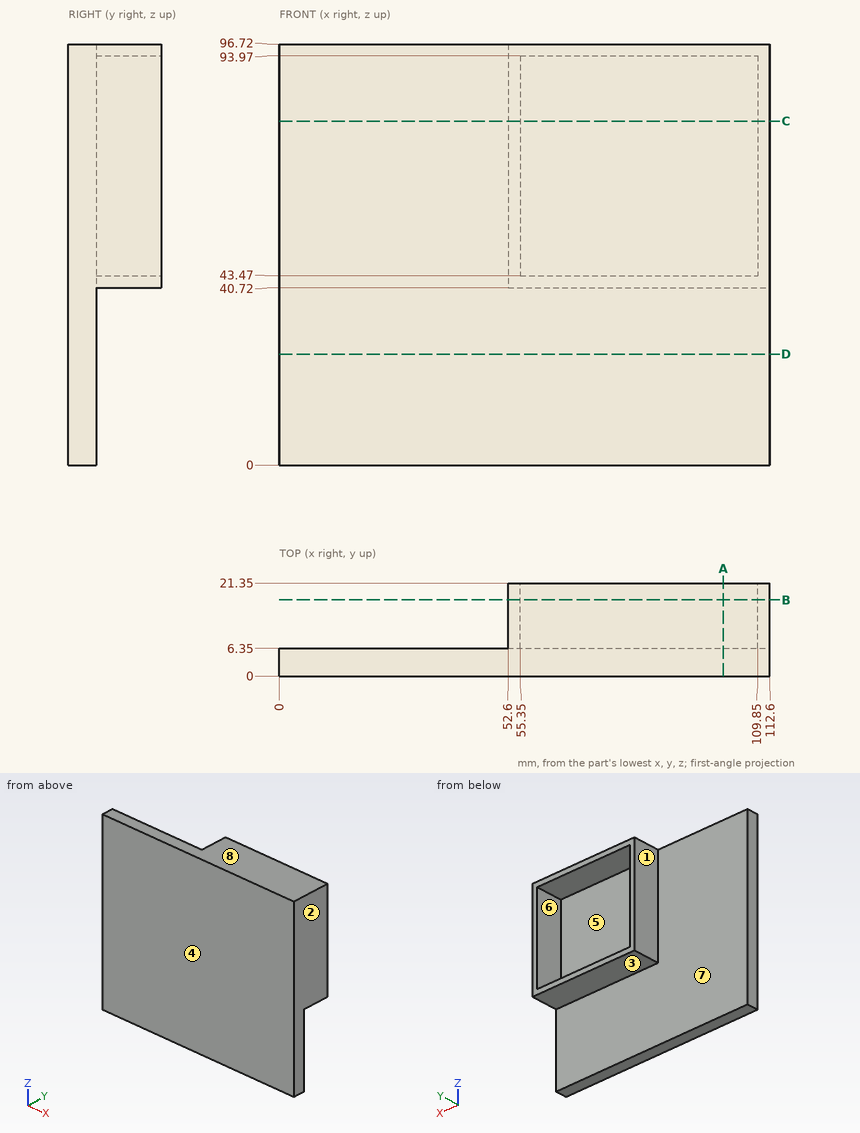
Can you work these out from the drawing? Everything is in mm from the part's minimum corner. A direction names the side the tool comes from. Give positions to 0.01 mm unless a question says otherwise; leave off trailing zeros. Loops run counter-clockwise (first coordinate to the right, second up) from the corner with the lowest first, then second, coordinate; pieces in that order, holes last. Notation, with made-up numbers: (-24, -37.75) -> (19, -37.75) arc R20 cw to (19, -12.75) -> close; hole circle Ø10 at (-10.5, 13.5). An arc over 180 degrees is marked (long way). Put each result on its own line as item: value.
(1) Thinking about a two-plate mould opening in Z: for the marked faces 6, 7 and 8, which applies, pulls with the +Z half, pulls with the -Z half, needs draft (parallel to the pull), parting line crosses it, or undercut?
Computed:
face 6: undercut
face 7: needs draft
face 8: pulls with the +Z half
(2) Please list where these lines run through material, in increasing order: probe 1 along X at (y, z) = (19.75, 90.5); probe 2 along Z at (x, y) = (60, 13.25); probe 3 along Y at (x, z) = (97, 76.5). Write a range as [from, to].
Computed:
probe 1: [52.6, 55.35], [109.85, 112.6]
probe 2: [40.72, 43.47], [93.97, 96.72]
probe 3: [0, 6.35]
(3) Imagine slicing it at B-B on y = 17.5. Write out the boundary of the cut face in (x, z), plus the area to 3 significant figures.
Computed:
outline: (52.6, 40.72) -> (112.6, 40.72) -> (112.6, 96.72) -> (52.6, 96.72) -> close; hole (55.35, 43.47) -> (109.85, 43.47) -> (109.85, 93.97) -> (55.35, 93.97) -> close
area: 608 mm^2
(4) I'm going to push flat-ended pins straight in: pin 1 Ø7.5 at (x, y) = (79, 11.5) entering from -Z; pin 2 Ø8 at (x, y) = (26, 10.5) entering from +Z; pin 3 Ø3 at (x, z) = (101, 72) entering from +Y; pin 4 Ø6 at (y, z) = (13.5, 38.5) entering from -X. Where does each tip first touch, or does it pass through?
Computed:
pin 1: z = 40.72
pin 2: through
pin 3: y = 6.35
pin 4: x = 52.6
(5) Imagine slicing it at A-A on x = 102. Write out the boundary of the cut face in (y, z).
Computed:
outline: (0, 0) -> (6.35, 0) -> (6.35, 40.72) -> (21.35, 40.72) -> (21.35, 43.47) -> (6.35, 43.47) -> (6.35, 93.97) -> (21.35, 93.97) -> (21.35, 96.72) -> (0, 96.72) -> close
(6) For the marked faces 1, 2, 3, 4 and 5, which set-ups out of +Z, -Z, +X, -X, +Y, -Y let a thin tool reach every point of the face, with its end or its side?
Computed:
face 1: +Z, -Z, -X, +Y
face 2: +Z, -Z, +X, +Y, -Y
face 3: -Z, +X, -X, +Y
face 4: +Z, -Z, +X, -X, -Y
face 5: +Y
(7) Imagine slicing it at C-C on z = 79. Write out the boundary of the cut face in (x, y).
Computed:
outline: (0, 0) -> (112.6, 0) -> (112.6, 21.35) -> (109.85, 21.35) -> (109.85, 6.35) -> (55.35, 6.35) -> (55.35, 21.35) -> (52.6, 21.35) -> (52.6, 6.35) -> (0, 6.35) -> close
(8) Imagine slicing it at D-D on z = 25.5. Write out the boundary of the cut face in (x, y), plus the area to 3 significant figures.
Computed:
outline: (0, 0) -> (112.6, 0) -> (112.6, 6.35) -> (0, 6.35) -> close
area: 715 mm^2
